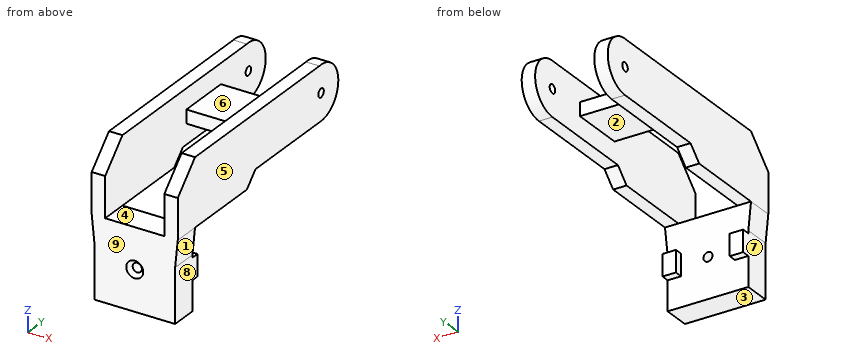
```python
from build123d import *

# Parameters (mm, degrees)
EXTRUDE_1_DEPTH     = 10
SKETCH_4_W          = 5
SKETCH_4_H          = 8
EXTRUDE_3_DEPTH     = 3
EXTRUDE_4_DEPTH     = 16
CUT_EXTRUDE_1_DEPTH = 11
SKETCH_15_W         = 5
SKETCH_15_H         = 20
EXTRUDE_5_DEPTH     = 22
OTHER_START         = -1
OTHER_4_OUTLINE_R   = 1.6
OTHER_4_DEPTH       = 32


# Read off the part's stored shape, not the designer's step: 高级异型孔3, 高级异型孔4
with BuildPart() as part:
    # 草图1 → 凸台-拉伸1 (new body)
    with BuildSketch(Plane(origin=(0, 0, 0), x_dir=(1, 0, 0), z_dir=(0, 1, 0))):
        Polygon((0, 10), (0, 30), (30, 30), (30, 10), (31, 0), (30, 0), (0, 0), (-1, 0), align=None)
    extrude(amount=-EXTRUDE_1_DEPTH)

    # 草图4 → 凸台-拉伸3 (add)
    with BuildSketch(Plane(origin=(0, 0, 0), x_dir=(1, 0, 0), z_dir=(0, 1, 0))):
        with Locations((2.5, 15)):
            Rectangle(SKETCH_4_W, SKETCH_4_H)
        with Locations((27.5, 15)):
            Rectangle(SKETCH_4_W, SKETCH_4_H)
    extrude(amount=EXTRUDE_3_DEPTH)

    # 高级异型孔3 outline → 高级异型孔3 (revolve, cut)
    with BuildSketch(Plane(origin=(15, 0, -15), x_dir=(1, 0, 0), z_dir=(0, 0, 1))):
        Polygon((0, -10), (3.15, -10), (1.7, -8.55), (1.7, 0), (0, 0), align=None)
    revolve(axis=Axis((15, 0, -15), (0, 1, 0)), mode=Mode.SUBTRACT)

    # 草图13 → 凸台-拉伸4 (add, symmetric)
    with BuildSketch(Plane(origin=(15, 0, 0), x_dir=(0, 0, -1), z_dir=(1, 0, 0))):
        with BuildLine():
            Line((-24.95762742, 72), (-24.95762742, 0))
            Line((-24.95762742, 0), (-14.95762742, -10))
            Line((-14.95762742, -10), (0, -10))
            Line((0, -10), (0, 30))
            Line((0, 30), (-5, 35))
            Line((-5, 35), (-5, 72.919595656))
            ThreePointArc((-5, 72.919595656), (-15.460285674, 82.908996895), (-24.95762742, 72))
        make_face()
    extrude(amount=EXTRUDE_4_DEPTH, both=True)

    # 草图13<2> → 切除-拉伸1 (cut, symmetric)
    with BuildSketch(Plane(origin=(15, 0, 0), x_dir=(0, 0, -1), z_dir=(1, 0, 0))):
        with BuildLine():
            Line((-24.95762742, 72), (-24.95762742, 0))
            Line((-24.95762742, 0), (-14.95762742, -10))
            Line((-14.95762742, -10), (0, -10))
            Line((0, -10), (0, 30))
            Line((0, 30), (-5, 35))
            Line((-5, 35), (-5, 72.919595656))
            ThreePointArc((-5, 72.919595656), (-15.460285674, 82.908996895), (-24.95762742, 72))
        make_face()
    extrude(amount=CUT_EXTRUDE_1_DEPTH, both=True, mode=Mode.SUBTRACT)

    # 草图15 → 凸台-拉伸5 (add)
    with BuildSketch(Plane(origin=(4, 0, 0), x_dir=(0, 0, -1), z_dir=(1, 0, 0))):
        with Locations((-14.95762742, 47)):
            Rectangle(SKETCH_15_W, SKETCH_15_H)
    extrude(amount=EXTRUDE_5_DEPTH)

    # 高级异型孔4 outline → 高级异型孔4 (cut)
    with BuildSketch(Plane.YZ.offset(OTHER_START)):
        with Locations((72.919595656, 15)):
            Circle(OTHER_4_OUTLINE_R)
    extrude(amount=OTHER_4_DEPTH, mode=Mode.SUBTRACT)


solid = part.part
```
Here's how the part is built. I have some questions about the finished solid (model axes, mm). Face numbers are marked on the shaded views. A direction names the side the tool comes from. Coordinates: 2 decimals unless noted, no trailing zeros. Order: outer loops, then holes, each group sorted by start corner. A loop starts at its lowest first (then second) coordinate and runs counter-clockwise, first axis right, second up. Notation, with made-up numbers: M -30.5,-25.5 L 27.5,-25.5 A24 cw 27.5,2.5 Z; hole C 5,-16.75 d5. An arc over 180 degrees is marked long. Answer as a JSON object with one key per item and string values. Group by question number.
(1) Suppose I cut it at B-B, the plane x = 15. Please give me the cut outline in (y, z).
(2) Which directions (+Z, -Z, +X, -X, +Y, -Y) give clear straight access to the entire face, cutting with the end or side of a thin tool? Please do the marked faces 5, 6, 7, 8 and 9.
(3) Suppose I cut it at D-D, the plane x = 20. Please give me the cut outline in (y, z).
(4) For pin 1 (2 mm diameter, centred on x = 2, y = 70, fed in from +Z); pin 2 (4 mm diameter, centred on x = 13.5, y = 47, fed in from +Z); pin 3 (0.9 mm diameter, centred on y = 1.5, z = -14.5, fed in from -X); pin 4 (1.9 mm diameter, centred on y = 72.92, z = 15, fed in from +X), each with a flat end and sliding along its axis, tell me the tip position at first contact or that it passes through.
(5) I need wall thicknesses on probe 1 along X at (y, z) = (-4, -15); probe 2 along X at (y, z) = (53, 12); probe 3 along Z at (x, y) = (15, -3.5). Which ranges of each line are inside material? Lowest first, please.
(6) If we mould it in two halves opening along X, with no side actions, what happens to the marked faces 1, 2, 3 and 4? For each: released by +X, released by -X, zero draft, split by the parting line, or undercut.
(7) Suppose I cut it at A-A, the plane z = -15. Please give me the cut outline in (x, y).
(8) Suppose I cut it at C-C, the plane y = 5.5. Please give me the cut outline in (x, z), then the cut area to 3 significant figures.
Values found:
{
 "1": {"outline": "M -10,-30 L 0,-30 L 0,-16.7 L -8.55,-16.7 L -10,-18.15 Z; M -10,-11.85 L -8.55,-13.3 L 0,-13.3 L 0,0 L -10,0 Z; M 37,12.46 L 57,12.46 L 57,17.46 L 37,17.46 Z"},
 "2": {"face 5": "+Z, -Z, +X, +Y, -Y", "face 6": "+Z, +Y, -Y", "face 7": "-Z, -X, +Y, -Y", "face 8": "-Z, +X, +Y, -Y", "face 9": "+Z, -Z, +X, -X, -Y"},
 "3": {"outline": "M -10,-30 L 0,-30 L 0,0 L -10,0 Z; M 37,12.46 L 57,12.46 L 57,17.46 L 37,17.46 Z"},
 "4": {"pin 1": "stops at z = 24.96", "pin 2": "stops at z = 17.46", "pin 3": "stops at x = 0", "pin 4": "passes through"},
 "5": {"probe 1": "x = 0 to 13.3, 16.7 to 30", "probe 2": "x = -1 to 4, 26 to 31", "probe 3": "z = -30 to -16.7, -13.3 to 0"},
 "6": {"face 1": "released by +X", "face 2": "undercut", "face 3": "zero draft", "face 4": "undercut"},
 "7": {"outline": "M 0,-10 L 11.85,-10 L 13.3,-8.55 L 13.3,0 L 5,0 L 5,3 L 0,3 Z; M 16.7,-8.55 L 18.15,-10 L 30,-10 L 30,3 L 25,3 L 25,0 L 16.7,0 Z"},
 "8": {"outline": "M -1,0 L 4,0 L 4,24.96 L -1,24.96 Z; M 26,0 L 31,0 L 31,24.96 L 26,24.96 Z", "area": "250 mm^2"}
}
